Work out the finished part from the listing and answer in its coordinate system (mm). Face numbers are marked on the shaded views. Round coordinates to 2 decimals unless told otherwise and drop trailing zeros. Use one line per item in the form item = value.
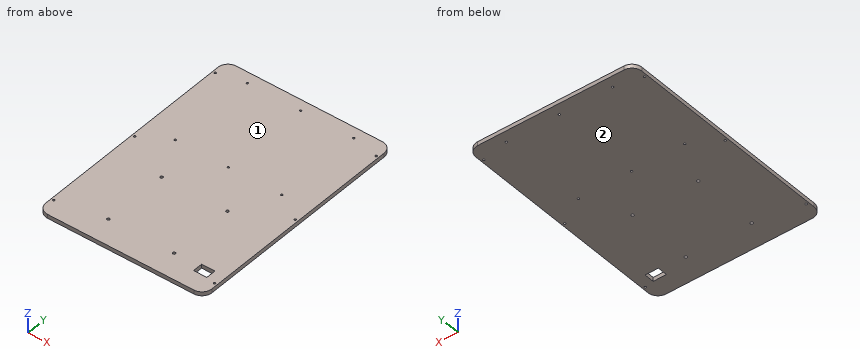
Autodesk Inventor part; units mm, degrees
ref_plane "YZ Plane" through (0, 0, 0) normal (1, 0, 0) x (0, 1, 0)
ref_plane "XZ Plane" through (0, 0, 0) normal (0, 1, 0) x (-1, 0, 0)
ref_plane "XY Plane" through (0, 0, 0) normal (0, 0, 1) x (1, 0, 0)
sketch "Sketch1" plane through (0, 0, 0) normal (0, 0, 1) x (1, 0, 0)
  line L0 (-125, -175) -> (125, -175)
  line L1 (125, -175) -> (125, 175)
  line L2 (125, 175) -> (-125, 175)
  line L3 (-125, 175) -> (-125, -175)
  line L4 (-125, -175) -> (125, 175) construction
  line L5 (125, -175) -> (-125, 175) construction
  line L6 (-121, -150) -> (121, -150)
  line L7 (121, -150) -> (121, 150)
  line L8 (121, 150) -> (-121, 150)
  line L9 (-121, 150) -> (-121, -150)
  line L10 (-121, -150) -> (121, 150) construction
  line L11 (121, -150) -> (-121, 150) construction
  circle A0 centre (121, 150) radius 1.5
  circle A1 centre (-121, 150) radius 1.5
  circle A2 centre (-121, -150) radius 1.5
  circle A3 centre (121, -150) radius 1.5
  circle A4 centre (-121, 0) radius 1.5
  circle A5 centre (121, 0) radius 1.5
  line L12 (0, 0) -> (0, -175)
  line L13 (-125, 0) -> (125, -175)
  line L14 (125, 0) -> (-125, -175)
  circle A6 centre (49.4975, -38.0025) radius 2.05
  circle A7 centre (-49.4975, -38.0025) radius 2.05
  circle A8 centre (49.4975, -136.9975) radius 2.05
  circle A9 centre (-49.4975, -136.9975) radius 2.05
  point P0 (121, -148.5)
  point P1 (119.5, -150)
  point P2 (119.5, 150)
  point P3 (121, 148.5)
  point P4 (-121, 148.5)
  point P5 (-119.5, 150)
  point P6 (0, -87.5)
  dimension "d0" = 250
  dimension "d1" = 350
  dimension "d10" = 242
  dimension "d11" = 300
  dimension "d12" = 3
  dimension "d13" = 3
  dimension "d14" = 3
  dimension "d15" = 3
  dimension "d16" = 3
  dimension "d17" = 3
  dimension "d24" = 4.1
  dimension "d25" = 4.1
  dimension "d26" = 4.1
  dimension "d27" = 4.1
extrude "Extrusion1" add sketch "Sketch1" along normal blind 6 contours L14 L6 L12 L0 | L3 L13 L9 A2 L6 L14 | L12 L6 L13 L0 | L3 L2 L1 L14 L7 A5 A0 L8 A1 L9 A4 L13 | L14 L12 L6 | L6 A2 L9 L13 L14 | L13 L6 A3 L7 L14 L1 | L12 L13 L6 | L9 A4 A1 L8 A0 L7 A5 L14 L13 | L14 L7 A3 L6 L13
fillet "Fillet1" radius 15 4 edges at (125, 175, 3) (125, -175, 3) (-125, -175, 3) (-125, 175, 3)
sketch "Sketch2" plane through (0, 0, 6) normal (0, 0, 1) x (1, 0, 0)
  line L0 (90, -127.5) -> (104.4, -127.5)
  line L1 (87.2, -127.5) -> (107.2, -127.5)
  line L2 (87.2, -127.5) -> (107.2, -127.5)
  line L3 (107.2, -127.5) -> (107.2, -147.5)
  line L4 (107.2, -147.5) -> (87.2, -147.5)
  line L5 (87.2, -147.5) -> (87.2, -127.5)
  line L6 (87.2, -147.5) -> (107.2, -147.5)
  line L7 (107.2, -147.5) -> (107.2, -132.5)
  line L8 (107.2, -132.5) -> (87.2, -132.5)
  line L9 (87.2, -132.5) -> (87.2, -147.5)
  point P0 (0, 0)
  point P1 (97.2, -127.5)
  dimension "d28" = 20
  dimension "d29" = 20
  dimension "d30" = 20
  dimension "d31" = 20
  dimension "d32" = 15
extrude "Extrusion2" cut sketch "Sketch2" against normal through all contours L8 L3 L4 L5
sketch "Sketch3" plane through (0, 0, 6) normal (0, 0, 1) x (1, 0, 0)
  circle A0 centre (80, 25) radius 1.5
  circle A1 centre (0, 25) radius 1.5
  circle A2 centre (-80, 25) radius 1.5
  circle A3 centre (-80, 159) radius 1.5
  circle A4 centre (0, 159) radius 1.5
  circle A5 centre (80, 159) radius 1.5
  point P0 (0, 0)
extrude "Extrusion3" cut sketch "Sketch3" against normal through all
properties part number "manipulation layer"
(1) Given P1, Ø1, axis at x = 80.5, y = 9.5, coming from the -Z side; P2, Ø2.5, axis at x = 49.5, y = -137, coming from the +Z side, each flat-ended and moving along its own axis, determine where each tip first touches the part or whether it passes through.
Completed:
P1 = 0
P2 = through
(2) Consider L1, parallel to Y at x = 0, z = 4.55; L2, parallel to X at y = 150, z = 3.4; L3, parallel to Y at x = 92.5, z = 3. Determine where each line is inside the solid, lowest interval first.
Completed:
L1 = -175 to 23.5, 26.5 to 157.5, 160.5 to 175
L2 = -125 to -122.5, -119.5 to 119.5, 122.5 to 125
L3 = -175 to -147.5, -132.5 to 175
(3) For a pull along Z with two mould halves and no side action, classify the marked faces 1 and 2 as +Z half, -Z half, draft (parallel to the pull), parting line (faces both ways), or undercut.
Completed:
face_1 = +Z half
face_2 = -Z half
